For this review, take the finished solid that the model builds, in its own axes (mm). A direction names the side the tool comes from. Coordinates: 2 decimals unless noted, no trailing zeros. Loops run counter-clockwise (first coordinate to the right, second up) from the corner with the lowest first, then second, coordinate; pieces in that order, holes last. Notation, with made-up numbers: (-22.75, 30.25) -> (-11.75, 30.25) arc R14 cw to (-11.75, 36.25) -> close; hole circle Ø4 at (18.5, 55). An arc over 180 degrees is marked (long way). Answer in a Markdown table with one row per item.
from build123d import *

# Parameters (mm, degrees)
F0_W     = 20
F0_H     = 20
F1_DEPTH = 40
F2_W     = 20
F2_H     = 20
F3_DEPTH = 20
F4_W     = 20
F4_H     = 20
F5_DEPTH = 40


with BuildPart() as f1:
    # F0 (on Front) → F1 (new body)
    with BuildSketch(Plane.XZ):
        with Locations((10, 10)):
            Rectangle(F0_W, F0_H)
    extrude(amount=F1_DEPTH)

    # F2 (on face) → F3 (join)
    with BuildSketch(Plane(origin=(0, 0, 0), x_dir=(1, 0, 0), z_dir=(0, 0, -1))):
        with Locations((10, 30)):
            Rectangle(F2_W, F2_H)
    extrude(amount=F3_DEPTH)

    # F4 (on face) → F5 (join)
    with BuildSketch(Plane.YZ.offset(20)):
        with Locations((-30, -10)):
            Rectangle(F4_W, F4_H)
    extrude(amount=F5_DEPTH)


solid = f1.part
Item 1: Insertion check: pin 1 (3 mm diameter, centred on x = 28.5, y = -17.5, fed in from +Z); pin 2 (1 mm diameter, centred on y = -10, z = 13, fed in from +X); pin 3 (10 mm diameter, centred on x = 44, z = -11, fed in from +Y). Each pin has a flat end and moves straight along its axis. Give the tip position at first contact, or say it passes through.
Worked answers:
| item | result |
|---|---|
| pin 1 | through |
| pin 2 | x = 20 |
| pin 3 | y = -20 |
Item 2: Take a section at D-D, the plane y = -8. State the section outline as (x, z) points, and give its area (3 significant figures).
Worked answers:
| item | result |
|---|---|
| outline | (0, 0) -> (20, 0) -> (20, 20) -> (0, 20) -> close |
| area | 400 mm² |
Item 3: Take a section at B-B, the plane z = 6. State the section outline as (x, y) points, and give its area (3 significant figures).
Worked answers:
| item | result |
|---|---|
| outline | (0, -40) -> (20, -40) -> (20, 0) -> (0, 0) -> close |
| area | 800 mm² |
Item 4: For faces 1 (the flat face through (10, -10, 0)), 2 (the flat face through (40, -30, 0)), 3 (the flat face through (10, -20, 20)), list the 3-axis set-ups (+Z, -Z, +X, -X, +Y, -Y) from which the entire face can be reached by the end or side of a thin tool; tool diameter is ignored.
Worked answers:
| item | result |
|---|---|
| face 1 | -Z, +X, -X, +Y |
| face 2 | +Z, +X, +Y, -Y |
| face 3 | +Z, +X, -X, +Y, -Y |
Item 5: For L1, parallel to Y at x = 36, z = -4.5; L2, parallel to Z at x = 23, y = -24.5; L3, parallel to X at y = -28, z = 4, list the stretches that pass through material, from the lowest coordinate up.
Worked answers:
| item | result |
|---|---|
| L1 | -40 to -20 |
| L2 | -20 to 0 |
| L3 | 0 to 20 |
Item 6: Take a section at A-A, the plane y = -27.5. State the section outline as (x, z) points.
Worked answers:
| item | result |
|---|---|
| outline | (0, -20) -> (60, -20) -> (60, 0) -> (20, 0) -> (20, 20) -> (0, 20) -> close |
Item 7: Take a section at C-C, the plane x = 4. State the section outline as (y, z) points.
Worked answers:
| item | result |
|---|---|
| outline | (-40, -20) -> (-20, -20) -> (-20, 0) -> (0, 0) -> (0, 20) -> (-40, 20) -> close |
